Source: three-view drawing plus pictorial views. Frame: mm from the lowest corner of the part. A direction names the side the tool comes from. Give positions to 0.01 mm unless a question says otherwise; leave off trailing zeros. Loops run counter-clockwise (first coordinate to the right, second up) from the corner with the lowest first, then second, coordinate; pieces in that order, holes last. Notation, with made-up numbers: M 35.5,20 L 88.5,20 A29 ccw 88.5,40 Z; hole C 12.25,77.5 d2. An arc over 180 degrees is marked long. One line per item, written item: value. Start each with the question number.
(1) Section A-A on x = 2. Output: boundary loops of the cut face in (y, z).
(2) Pin query (flat end, axial travel): P1, Ø3, axis at x = 18.45, z = 25.42, coming from the -Y side; P2, Ø8, axis at x = 4, y = 22, coming from the +Z side (1 decimal); P3, Ø5, axis at x = 17, z = 24.5, coming from the -Y side; P4, Ø1.5, axis at x = 15, y = 6, coming from the +Z side. Return the tip coordinate at first contact, or that it passes through.
(3) Section C-C on x = 4.5. Output: boundary loops of the cut face in (y, z) (1 decimal).
(4) Section B-B on z = 25. Output: boundary loops of the cut face in (x, y) (1 decimal).
(5) Ray query, line 1 along Y through (x, z) = (9.5, 5.25); line 2 along Y through (x, z) = (17.75, 20.25); line 3 along X through (y, z) = (4.5, 25.75) (1 decimal). Return the intervals inside material, ascending. Write a range as from..to.
(6) Access query for the marked faces 1, 2, 3, 4 and 5. Directions: +Z, -Z, +X, -X, +Y, -Y. A direction counts if a zero-diameter tool reaches every point of the face in a straight line with its end or side. Return the directions, or none.
(7) Pull-direction query (Z, two-part tool) for the marked faces 6, 7 and 8; classes: released by +Z, released by -Z, zero draft, split by the parting line, or undercut.
(8) Section D-D on z = 7. Output: boundary loops of the cut face in (x, y).
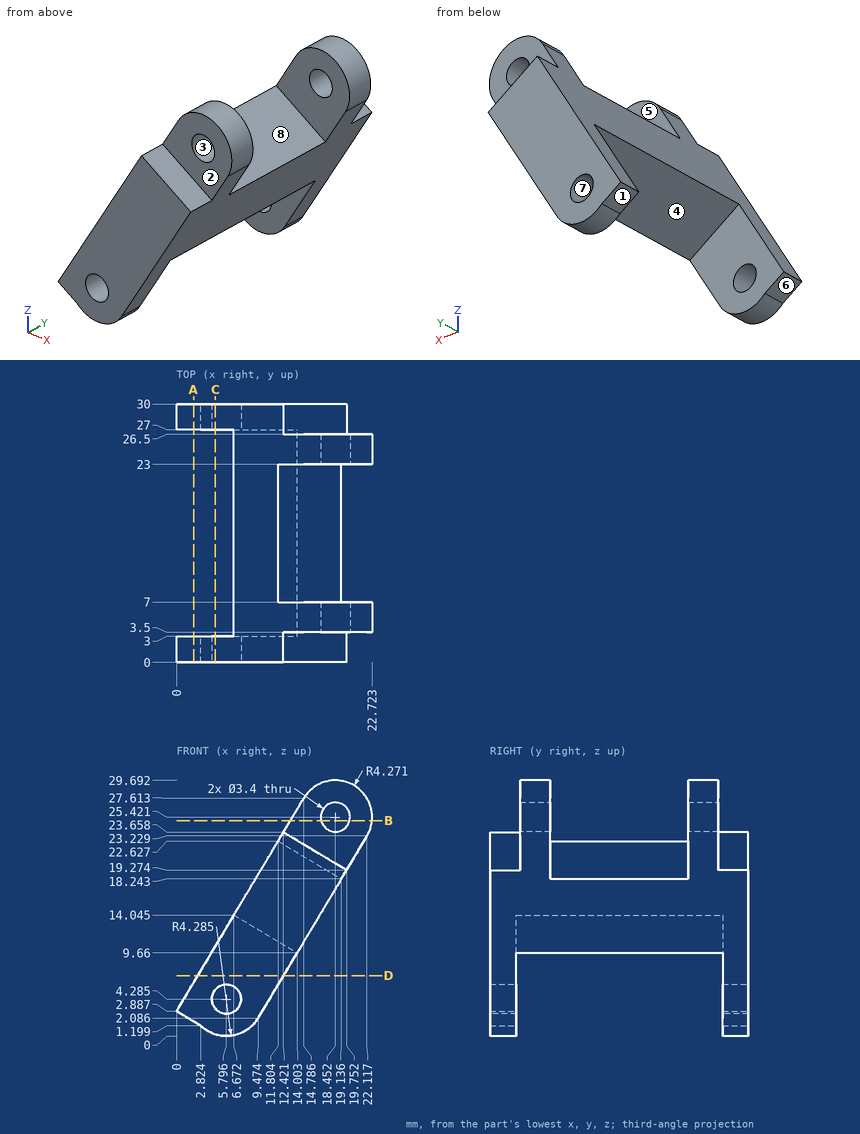
Output values:
1. outline: M 0,1.69 L 3,1.69 L 3,6.23 L 0,6.23 Z; M 27,1.69 L 30,1.69 L 30,6.23 L 27,6.23 Z
2. P1: passes through
2. P2: stops at z = 16.3
2. P3: stops at y = 3.5
2. P4: stops at z = 28.73
3. outline: M 0,0.2 L 3,0.2 L 3,3.2 L 0,3.2 Z; M 0,5.4 L 3,5.4 L 3,10.4 L 0,10.4 Z; M 27,0.2 L 30,0.2 L 30,3.2 L 27,3.2 Z; M 27,5.4 L 30,5.4 L 30,10.4 L 27,10.4 Z
4. outline: M 13.2,3.5 L 16.8,3.5 L 16.8,7 L 13.2,7 Z; M 13.2,23 L 16.8,23 L 16.8,26.5 L 13.2,26.5 Z; M 20.1,3.5 L 22.7,3.5 L 22.7,7 L 20.1,7 Z; M 20.1,23 L 22.7,23 L 22.7,26.5 L 20.1,26.5 Z
5. line 1: y = 0..3, 27..30
5. line 2: y = 0..7, 23..30
5. line 3: x = 13.7..16.8, 20.1..22.7
6. face 1: -Z, -X, +Y, -Y
6. face 2: +Z, +X, -Y
6. face 3: +Y, -Y
6. face 4: -Z, -X
6. face 5: +Z, +X
7. face 6: released by -Z
7. face 7: undercut
7. face 8: released by +Z
8. outline: M 2.46,0 L 12.41,0 L 12.41,3 L 2.46,3 Z; M 2.46,27 L 12.41,27 L 12.41,30 L 2.46,30 Z
